Study the drawing (mm; zero at the part's minimum x, y, z) and answer. A direction names the side the tool comes from. Coordinates: 2 decimals unless noted, no trailing zeros. Order: outer loops, then holes, each group sorted by start corner. A loop starts at its lowest first (then second) coordinate and runs counter-clockwise, first axis right, second up. Notation, with made-up numbers: M 7,3 L 59,3 A9 ccw 59,20 Z; hole C 45,78.25 d5. An arc over 180 degrees is marked long. One line per item, written item: value. Start each with the question number.
Q1. The part is cut by section B-B on y = 3.25. Give the vertices of the cut face in (x, z) (3 decimals), then the cut area to 3 significant figures.
Q2. The part is cut by section C-C on x = 2.54. Give the vertices of the cut face in (y, z) (3 decimals).
Q3. Determine the mould class of the marked faces 1, 2 and 3 for opening direction X: pulls with the +X half, pulls with the -X half, needs draft (parallel to the pull), parting line crosses it, or undercut.
Q4. Straight lines are drawn through the part: line 1 along X through (y, z) = (2.25, 8.5); line 2 along X through (y, z) = (0.85, 19.05); line 3 along X through (y, z) = (7.75, 12.5). For each, find the intervals that lie inside material, in ascending order. Write a range as [from, to].
Q5. Each of these flat-tipped pins is pushed along its axis until it touches: pin 1 Ø2 at (x, y) = (30.5, 3.5) entering from +Z (3 decimals); pin 2 Ø5 at (x, y) = (8, 4.5) entering from +Z (3 decimals); pin 3 Ø3.5 at (x, z) = (29, 11.5) entering from +Y. Where does it stop, or does it pass through?
Q6. The part is cut by section D-D on y = 1.25. Give the vertices of the cut face in (x, z).
Q7. The part is cut by section A-A on z = 2.54. Give the vertices of the cut face in (x, y).
Q8. For the marked faces 4, 5, 6 and 7, determine the directions among +Z, -Z, +X, -X, +Y, -Y from which every point of the face is accessible in a straight line to the end or side of a thin tool.
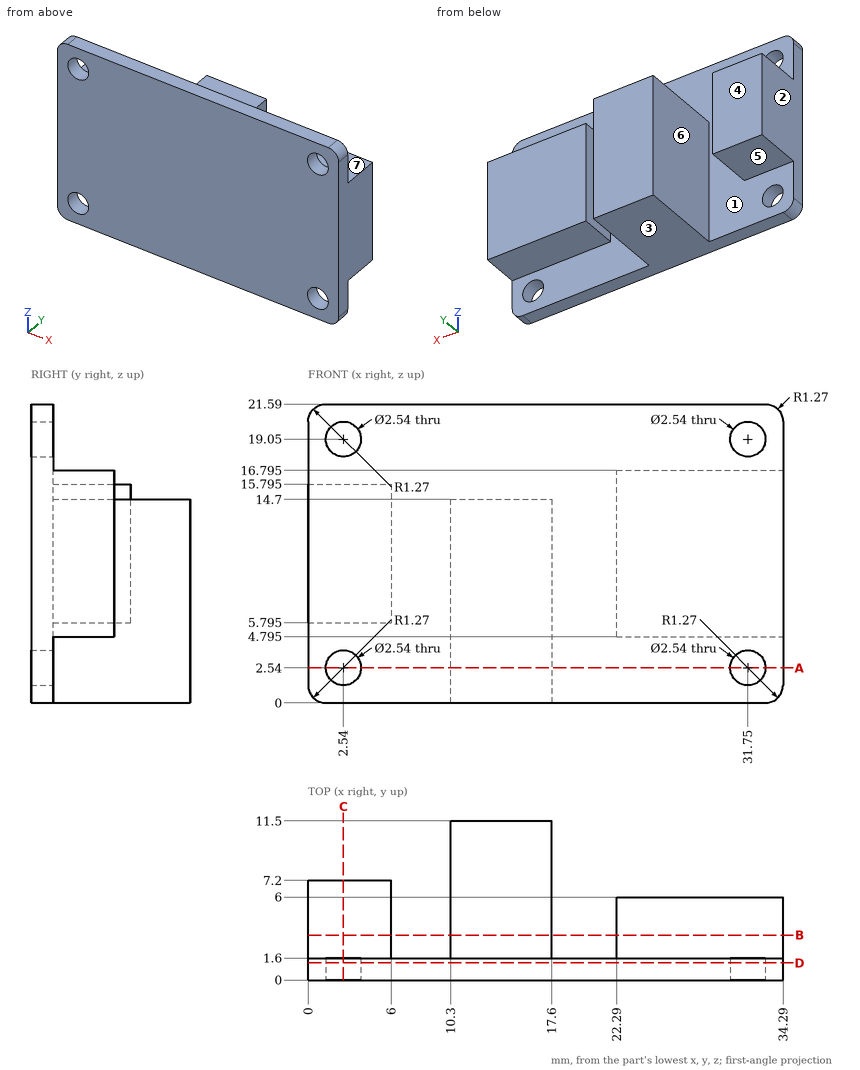
Output:
1. outline: M 0,5.795 L 6,5.795 L 6,15.795 L 0,15.795 Z; M 10.3,0 L 17.6,0 L 17.6,14.7 L 10.3,14.7 Z; M 22.29,4.795 L 34.29,4.795 L 34.29,16.795 L 22.29,16.795 Z
1. area: 311 mm^2
2. outline: M 0,0 L 1.6,0 L 1.6,1.27 L 0,1.27 Z; M 0,3.81 L 1.6,3.81 L 1.6,5.795 L 7.2,5.795 L 7.2,15.795 L 1.6,15.795 L 1.6,17.78 L 0,17.78 Z; M 0,20.32 L 1.6,20.32 L 1.6,21.59 L 0,21.59 Z
3. face 1: undercut
3. face 2: pulls with the -X half
3. face 3: needs draft
4. line 1: x = [0, 6], [10.3, 17.6], [22.29, 34.29]
4. line 2: x = [0, 1.27], [3.81, 30.48], [33.02, 34.29]
4. line 3: x = [10.3, 17.6]
5. pin 1: stops at z = 16.795
5. pin 2: stops at z = 15.795
5. pin 3: stops at y = 6
6. outline: M 0,1.27 A1.27 ccw 1.27,0 L 33.02,0 A1.27 ccw 34.29,1.27 L 34.29,20.32 A1.27 ccw 33.02,21.59 L 1.27,21.59 A1.27 ccw 0,20.32 Z; hole C 2.54,2.54 d2.54; hole C 2.54,19.05 d2.54; hole C 31.75,2.54 d2.54; hole C 31.75,19.05 d2.54
7. outline: M 0,0 L 1.27,0 L 1.27,1.6 L 0,1.6 Z; M 3.81,0 L 30.48,0 L 30.48,1.6 L 17.6,1.6 L 17.6,11.5 L 10.3,11.5 L 10.3,1.6 L 3.81,1.6 Z; M 33.02,0 L 34.29,0 L 34.29,1.6 L 33.02,1.6 Z
8. face 4: +Z, -Z, -X, +Y
8. face 5: -Z, -X, +Y
8. face 6: +Z, -Z, +Y
8. face 7: +Z, +X, -X, +Y
